```python
from build123d import *

# Parameters (mm, degrees)
F0_W     = 40
F0_H     = 30
F1_DEPTH = 25
F2_R     = 9.873161
F3_DEPTH = 10
F4_R     = 6
F5_DEPTH = 25
F7_DEPTH = 40


with BuildPart() as f1:
    # F0 (on Top) → F1 (new body)
    with BuildSketch(Plane.XY):
        with Locations((6.881981, 0)):
            Rectangle(F0_W, F0_H)
    extrude(amount=F1_DEPTH)

    # F2 (on face) → F3 (cut)
    with BuildSketch(Plane(origin=(0, 0, 0), x_dir=(1, 0, 0), z_dir=(0, 0, -1))):
        with Locations((9.873161, 0)):
            Circle(F2_R)
    extrude(amount=-F3_DEPTH, mode=Mode.SUBTRACT)

    # F4 (on face) → F5 (cut)
    with BuildSketch(Plane(origin=(0, 0, 10), x_dir=(1, 0, 0), z_dir=(0, 0, -1))):
        with Locations((9.873161, 0)):
            Circle(F4_R)
    extrude(amount=-F5_DEPTH, mode=Mode.SUBTRACT)

    # F6 (on face) → F7 (join)
    with BuildSketch(Plane(origin=(-13.118019, 0, 0), x_dir=(0, -1, 0), z_dir=(-1, 0, 0))):
        with BuildLine():
            ThreePointArc((-2.117814, 6.992008), (2.871889, 7.40042), (5.256141, 11.802609))
            ThreePointArc((5.256141, 11.802609), (2.376464, 16.490832), (-3.107196, 16.04199))
            ThreePointArc((-3.107196, 16.04199), (-0.82282, 14.103278), (0.031131, 11.231389))
            ThreePointArc((0.031131, 11.231389), (-0.536786, 8.854926), (-2.117814, 6.992008))
        make_face()
    extrude(amount=F7_DEPTH)


solid = f1.part
```
Source: CAD feature listing. Evaluate the final solid. Frame: model axes, mm. A direction names the side the tool comes from. Coordinates: 2 decimals unless noted, no trailing zeros. Order: outer loops, then holes, each group sorted by start corner. A loop starts at its lowest first (then second) coordinate and runs counter-clockwise, first axis right, second up. Notation, with made-up numbers: (21.25, 36.25) - (54.25, 36.25) arc R24 cw to (54.25, 47.25) - close; hole circle Ø11 at (2, 37.5). An arc over 180 degrees is marked (long way). One line per item, written item: value.
1) Mould query, pull axis X, two halves, no side actions, for faces 3 (the face through (-13.118, 3, 12)), 4 (the face through (19.29, -2.97, 4.93)), 5 (the face through (7, -15, 12)). Classes: released by +X, released by -X, zero draft, split by the parting line, or undercut.
Computed values:
face 3: released by -X
face 4: undercut
face 5: zero draft
2) Cut plane B-B on z = 5. Output: boundary loops of the cut face in (x, y).
Computed values:
outline: (-13.12, -15) - (26.88, -15) - (26.88, 15) - (-13.12, 15) - close; hole circle Ø19.75 at (9.87, 0)
3) Cut plane D-D on y = 9. Output: boundary loops of the cut face in (x, z).
Computed values:
outline: (-13.12, 0) - (5.81, 0) - (5.81, 10) - (13.93, 10) - (13.93, 0) - (26.88, 0) - (26.88, 25) - (-13.12, 25) - close
4) Cut plane A-A on y = -3.5. Output: boundary loops of the cut face in (x, z).
Computed values:
outline: (-53.12, 7.88) - (-13.12, 7.88) - (-13.12, 0) - (0.64, 0) - (0.64, 10) - (5, 10) - (5, 25) - (-13.12, 25) - (-13.12, 15.72) - (-53.12, 15.72) - close; (14.75, 10) - (19.11, 10) - (19.11, 0) - (26.88, 0) - (26.88, 25) - (14.75, 25) - close
5) Contact query for flat-ended pins moving along their axis: pin 1 (6 mm diameter, centred on x = 10.5, y = 0, fed in from -Z); pin 2 (3 mm diameter, centred on x = -20, z = 18, fed in from -Y); pin 3 (4 mm diameter, centred on y = 6, z = 21.5, fed in from -X); pin 4 (12 mm diameter, centred on x = -44.5, y = 3, fed in from -Z). Output: stop coordinate, or through.
Computed values:
pin 1: passes through
pin 2: stops at y = -2.36
pin 3: stops at x = -13.12
pin 4: stops at z = 6.55
6) Reachability of faces 1 (the face through (15.416, 2.298, 17.395)), 2 (the face through (16.3, -0.1, 10)) from +Z, -Z, +X, -X, +Y, -Y: full face, straight path, thin tool, end or side. Return the list, or none.
Computed values:
face 1: +Z, -Z
face 2: -Z
7) Ray query, line 1 (X direction, y = 0, z = 2); line 2 (Z direction, x = 16.5, y = 4.25); line 3 (X direction, y = 0, z = 18.25). Return the intervals inside material, ascending. Write a range as [from, to].
Computed values:
line 1: x = [-13.12, 0], [19.75, 26.88]
line 2: z = [10, 25]
line 3: x = [-13.12, 3.87], [15.87, 26.88]
8) Cut plane C-C on x = -23. Output: boundary loops of the cut face in (y, z) (3 decimals), plus the area to 3 significant figures.
Computed values:
outline: (-0.031, 11.231) arc R5.256 cw to (3.107, 16.042) arc R5.256 ccw (long way) to (2.118, 6.992) arc R5.256 cw to start
area: 52.9 mm^2
